Input: part model. Units: mm. Frame: model coordinates. Give positions to 0.01 mm unless a question says otherwise; leave off trailing zeros. Write each loop counter-clockwise with the first axis right and the second up, starting at its lowest first coordinate (ties: lowest second). Pieces come first, ordered by that corner, then holes. Notation, with made-up numbers: (-4.5, 48.25) -> (28.5, 48.25) arc R9 cw to (28.5, 52.25) -> close; hole circle Ø4 at (75, 80). An arc over 180 degrees is marked (long way). Return JSON: item names as keys, results as strings. Group by question number.
Item 1: Section A-A, the plane y = 0. Return loops of the section in (x, z), then the cut area to 3 significant figures.
Item 2: Line query: line 1 (X direction, y = 9, z = 422); line 2 (Y direction, x = 5.5, z = 549); line 3 (Y direction, x = -14, z = 414). Output: solid intervals per line, ascending. Write a range as [from, to].
Item 3: Pin query (flat end, axial travel): P1, Ø10, axis at x = 12.5, y = -9, coming from the +Z side; P2, Ø0.8, axis at y = 17, z = 523.5, coming from the -X side; P3, Ø0.8, axis at y = -17, z = 550, coming from the +X side; P4, Ø1.1, axis at x = 0.5, z = 474.5, coming from the +Y side. Return the tip coordinate at first contact, or that it passes through.
from build123d import *

# Parameters (mm, degrees)
SKETCH1_R               = 3.3274
BOSS_EXTRUDE1_DEPTH     = 609.6
SKETCH2_W               = 42.839593621
SKETCH2_H               = 1002.279512573
CUT_EXTRUDE1_DEPTH      = 5.334
CUT_EXTRUDE1_DEPTH_BACK = 41.148


with BuildPart() as part:
    # Sketch1 → Boss-Extrude1 (new body, symmetric)
    with BuildSketch(Plane.XY):
        with BuildLine():
            Line((-10.287, 13.552357131), (-10.287, 14.0843))
            ThreePointArc((-10.287, 14.0843), (-10.022898185, 14.721898185), (-9.3853, 14.986))
            Line((-9.3853, 14.986), (-5.617617549, 14.986))
            ThreePointArc((-5.617617549, 14.986), (-4.519044045, 15.441044045), (-4.064, 16.539617549))
            Line((-4.064, 16.539617549), (-4.064, 17.496382451))
            ThreePointArc((-4.064, 17.496382451), (-4.519044045, 18.594955955), (-5.617617549, 19.05))
            Line((-5.617617549, 19.05), (-7.974178704, 19.05))
            ThreePointArc((-7.974178704, 19.05), (-8.736178704, 18.288), (-9.498178704, 19.05))
            Line((-9.498178704, 19.05), (-14.327719207, 19.05))
            ThreePointArc((-14.327719207, 19.05), (-15.087603123, 18.231251131), (-15.847487039, 19.05))
            ThreePointArc((-15.847487039, 19.05), (-18.120176289, 18.120192083), (-19.05, 15.847509295))
            ThreePointArc((-19.05, 15.847509295), (-18.231250992, 15.08762539), (-19.05, 14.327741484))
            Line((-19.05, 14.327741484), (-19.05, 9.496091471))
            ThreePointArc((-19.05, 9.496091471), (-18.231250992, 8.736207565), (-19.05, 7.97632366))
            Line((-19.05, 7.97632366), (-19.05, 5.617617549))
            ThreePointArc((-19.05, 5.617617549), (-18.594955955, 4.519044045), (-17.496382451, 4.064))
            Line((-17.496382451, 4.064), (-16.539617549, 4.064))
            ThreePointArc((-16.539617549, 4.064), (-15.441044045, 4.519044045), (-14.986, 5.617617549))
            Line((-14.986, 5.617617549), (-14.986, 9.385342516))
            ThreePointArc((-14.986, 9.385342516), (-14.721898185, 10.022940701), (-14.0843, 10.287042516))
            Line((-14.0843, 10.287042516), (-13.516042086, 10.287042516))
            ThreePointArc((-13.516042086, 10.287042516), (-13.170975923, 10.218404478), (-12.878443117, 10.022939917))
            Line((-12.878443117, 10.022939917), (-8.14758008, 5.292065243))
            ThreePointArc((-8.14758008, 5.292065243), (-7.117955879, 3.751120653), (-6.7564, 1.933453584))
            Line((-6.7564, 1.933453584), (-6.7564, -1.933453584))
            ThreePointArc((-6.7564, -1.933453584), (-7.117955879, -3.751120653), (-8.14758008, -5.292065243))
            Line((-8.14758008, -5.292065243), (-12.878443117, -10.022939917))
            ThreePointArc((-12.878443117, -10.022939917), (-13.170975923, -10.218404478), (-13.516042086, -10.287042516))
            Line((-13.516042086, -10.287042516), (-14.0843, -10.287042516))
            ThreePointArc((-14.0843, -10.287042516), (-14.721898185, -10.022940701), (-14.986, -9.385342516))
            Line((-14.986, -9.385342516), (-14.986, -5.617617549))
            ThreePointArc((-14.986, -5.617617549), (-15.441044045, -4.519044045), (-16.539617549, -4.064))
            Line((-16.539617549, -4.064), (-17.496382451, -4.064))
            ThreePointArc((-17.496382451, -4.064), (-18.594955955, -4.519044045), (-19.05, -5.617617549))
            Line((-19.05, -5.617617549), (-19.05, -7.976318491))
            ThreePointArc((-19.05, -7.976318491), (-18.231250992, -8.736202396), (-19.05, -9.496086302))
            Line((-19.05, -9.496086302), (-19.05, -14.32774291))
            ThreePointArc((-19.05, -14.32774291), (-18.231250992, -15.087626816), (-19.05, -15.847510721))
            ThreePointArc((-19.05, -15.847510721), (-18.120175716, -18.120192644), (-15.847486868, -19.05))
            ThreePointArc((-15.847486868, -19.05), (-15.087602952, -18.231251131), (-14.327719036, -19.05))
            Line((-14.327719036, -19.05), (-9.496062448, -19.05))
            ThreePointArc((-9.496062448, -19.05), (-8.736178532, -18.231251131), (-7.976294616, -19.05))
            Line((-7.976294616, -19.05), (-5.617617549, -19.05))
            ThreePointArc((-5.617617549, -19.05), (-4.519044045, -18.594955955), (-4.064, -17.496382451))
            Line((-4.064, -17.496382451), (-4.064, -16.539617549))
            ThreePointArc((-4.064, -16.539617549), (-4.519044045, -15.441044045), (-5.617617549, -14.986))
            Line((-5.617617549, -14.986), (-9.3853, -14.986))
            ThreePointArc((-9.3853, -14.986), (-10.022898185, -14.721898185), (-10.287, -14.0843))
            Line((-10.287, -14.0843), (-10.287, -13.552357131))
            ThreePointArc((-10.287, -13.552357131), (-10.218362387, -13.207291992), (-10.022898969, -12.91475973))
            Line((-10.022898969, -12.91475973), (-5.252158105, -8.144007132))
            ThreePointArc((-5.252158105, -8.144007132), (-3.715177372, -7.117027388), (-1.902183975, -6.7564))
            Line((-1.902183975, -6.7564), (1.902183975, -6.7564))
            ThreePointArc((1.902183975, -6.7564), (3.715177372, -7.117027388), (5.252158105, -8.144007132))
            Line((5.252158105, -8.144007132), (10.022898969, -12.91475973))
            ThreePointArc((10.022898969, -12.91475973), (10.218362387, -13.207291992), (10.287, -13.552357131))
            Line((10.287, -13.552357131), (10.287, -14.0843))
            ThreePointArc((10.287, -14.0843), (10.022898185, -14.721898185), (9.3853, -14.986))
            Line((9.3853, -14.986), (5.617617549, -14.986))
            ThreePointArc((5.617617549, -14.986), (4.519044045, -15.441044045), (4.064, -16.539617549))
            Line((4.064, -16.539617549), (4.064, -17.496382451))
            ThreePointArc((4.064, -17.496382451), (4.519044045, -18.594955955), (5.617617549, -19.05))
            Line((5.617617549, -19.05), (7.976294616, -19.05))
            ThreePointArc((7.976294616, -19.05), (8.736178532, -18.231251131), (9.496062448, -19.05))
            Line((9.496062448, -19.05), (14.327719036, -19.05))
            ThreePointArc((14.327719036, -19.05), (15.087602952, -18.231251131), (15.847486868, -19.05))
            ThreePointArc((15.847486868, -19.05), (18.120175716, -18.120192644), (19.05, -15.847510721))
            ThreePointArc((19.05, -15.847510721), (18.231250992, -15.087626816), (19.05, -14.32774291))
            Line((19.05, -14.32774291), (19.05, -9.496086302))
            ThreePointArc((19.05, -9.496086302), (18.231250992, -8.736202396), (19.05, -7.976318491))
            Line((19.05, -7.976318491), (19.05, -5.617617549))
            ThreePointArc((19.05, -5.617617549), (18.594955955, -4.519044045), (17.496382451, -4.064))
            Line((17.496382451, -4.064), (16.539617549, -4.064))
            ThreePointArc((16.539617549, -4.064), (15.441044045, -4.519044045), (14.986, -5.617617549))
            Line((14.986, -5.617617549), (14.986, -9.385342516))
            ThreePointArc((14.986, -9.385342516), (14.721898185, -10.022940701), (14.0843, -10.287042516))
            Line((14.0843, -10.287042516), (13.516042086, -10.287042516))
            ThreePointArc((13.516042086, -10.287042516), (13.170975923, -10.218404478), (12.878443117, -10.022939917))
            Line((12.878443117, -10.022939917), (8.14758008, -5.292065243))
            ThreePointArc((8.14758008, -5.292065243), (7.117955879, -3.751120653), (6.7564, -1.933453584))
            Line((6.7564, -1.933453584), (6.7564, 1.933453584))
            ThreePointArc((6.7564, 1.933453584), (7.117955879, 3.751120653), (8.14758008, 5.292065243))
            Line((8.14758008, 5.292065243), (12.878443117, 10.022939917))
            ThreePointArc((12.878443117, 10.022939917), (13.170975923, 10.218404478), (13.516042086, 10.287042516))
            Line((13.516042086, 10.287042516), (14.0843, 10.287042516))
            ThreePointArc((14.0843, 10.287042516), (14.721898185, 10.022940701), (14.986, 9.385342516))
            Line((14.986, 9.385342516), (14.986, 5.617617549))
            ThreePointArc((14.986, 5.617617549), (15.441044045, 4.519044045), (16.539617549, 4.064))
            Line((16.539617549, 4.064), (17.496382451, 4.064))
            ThreePointArc((17.496382451, 4.064), (18.594955955, 4.519044045), (19.05, 5.617617549))
            Line((19.05, 5.617617549), (19.05, 7.97632366))
            ThreePointArc((19.05, 7.97632366), (18.231250992, 8.736207565), (19.05, 9.496091471))
            Line((19.05, 9.496091471), (19.05, 14.327741484))
            ThreePointArc((19.05, 14.327741484), (18.231250992, 15.08762539), (19.05, 15.847509295))
            ThreePointArc((19.05, 15.847509295), (18.120176289, 18.120192083), (15.847487039, 19.05))
            ThreePointArc((15.847487039, 19.05), (15.087603123, 18.231251131), (14.327719207, 19.05))
            Line((14.327719207, 19.05), (9.498178704, 19.05))
            ThreePointArc((9.498178704, 19.05), (8.736178704, 18.288), (7.974178704, 19.05))
            Line((7.974178704, 19.05), (5.617617549, 19.05))
            ThreePointArc((5.617617549, 19.05), (4.519044045, 18.594955955), (4.064, 17.496382451))
            Line((4.064, 17.496382451), (4.064, 16.539617549))
            ThreePointArc((4.064, 16.539617549), (4.519044045, 15.441044045), (5.617617549, 14.986))
            Line((5.617617549, 14.986), (9.3853, 14.986))
            ThreePointArc((9.3853, 14.986), (10.022898185, 14.721898185), (10.287, 14.0843))
            Line((10.287, 14.0843), (10.287, 13.552357131))
            ThreePointArc((10.287, 13.552357131), (10.218362387, 13.207291992), (10.022898969, 12.91475973))
            Line((10.022898969, 12.91475973), (5.252158105, 8.144007132))
            ThreePointArc((5.252158105, 8.144007132), (3.715177372, 7.117027388), (1.902183975, 6.7564))
            Line((1.902183975, 6.7564), (-1.902183975, 6.7564))
            ThreePointArc((-1.902183975, 6.7564), (-3.715177372, 7.117027388), (-5.252158105, 8.144007132))
            Line((-5.252158105, 8.144007132), (-10.022898969, 12.91475973))
            ThreePointArc((-10.022898969, 12.91475973), (-10.218362387, 13.207291992), (-10.287, 13.552357131))
        make_face()
        Circle(SKETCH1_R, mode=Mode.SUBTRACT)
    extrude(amount=BOSS_EXTRUDE1_DEPTH, both=True)

    # Sketch2 → Cut-Extrude1 (cut, two sides)
    with BuildSketch(Plane(origin=(0, 19.05, 0), x_dir=(1, 0, 0), z_dir=(0, 1, 0))) as cut_extrude1_sk:
        with Locations((0.328899923, 110.810732084)):
            Rectangle(SKETCH2_W, SKETCH2_H)
    extrude(amount=CUT_EXTRUDE1_DEPTH, mode=Mode.SUBTRACT)
    extrude(cut_extrude1_sk.sketch, amount=-CUT_EXTRUDE1_DEPTH_BACK, mode=Mode.SUBTRACT)


solid = part.part
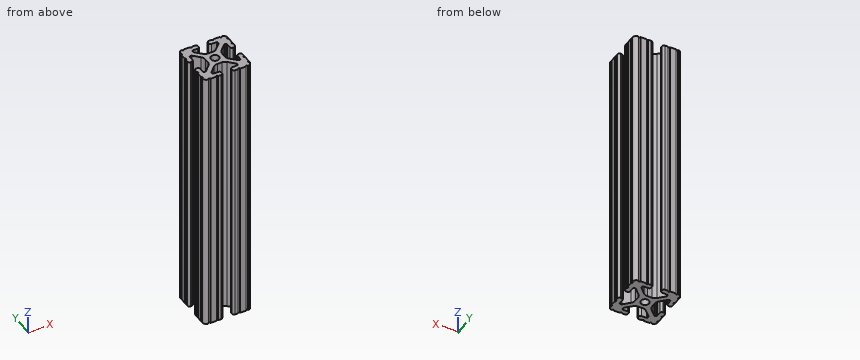
Answer below:
{
 "1": {"outline": "(-6.76, 390.33) -> (-3.33, 390.33) -> (-3.33, 609.6) -> (-6.76, 609.6) -> close; (3.33, 390.33) -> (6.76, 390.33) -> (6.76, 609.6) -> (3.33, 609.6) -> close", "area": "1,500 mm2"},
 "2": {"line 1": "x = [-18.28, -14.99], [-11.86, -6.11], [6.11, 11.86], [14.99, 18.28]", "line 2": "y = [-19.05, -14.99], [-8.39, 8.39], [14.99, 19.05]", "line 3": "y = [-19.05, -10.29], [10.29, 19.05]"},
 "3": {"P1": "stops at z = 609.6", "P2": "stops at x = -18.97", "P3": "stops at x = 18.97", "P4": "stops at y = 6.76"}
}
